Design review of the part built by this model. Coordinates are the model's own, in mm. A direction names the side the tool comes from. Coordinates: 2 decimals unless noted, no trailing zeros. Loops run counter-clockwise (first coordinate to the right, second up) from the corner with the lowest first, then second, coordinate; pieces in that order, holes last. Notation, with made-up numbers: (16.5, 39.5) - (71.5, 39.5) arc R32 cw to (71.5, 72.5) - close; hole circle Ø2 at (20, -33.75). An arc over 180 degrees is marked (long way). Answer in a Markdown table with one row per item. Add a question column.
(1) The part is to be moulded in two halves that separate along X. For faces 1 (the face through (-6.6, 24.02, -18.25)), 2 (the face through (-3.792, 14, -18)), 3 (the face through (-4, 28.312, -4)), say which applies: released by +X, released by -X, zero draft, split by the parting line, or undercut.
(2) We need section A-A, the plane y = 43. Write out the cut boundary in (x, z).
(3) We need section C-C, the plane x = 27.5. Write out the cut boundary in (y, z), plus the area to 3 significant figures.
(4) To check wall thickness, follow L1, parallel to X at y = 29, z = -18; L2, parallel to Z at x = 107, y = 11; L3, parallel to X at y = 46, z = -14. State the ranges of each line that lie inside material, in increasing order. Write a range as [from, to].
(5) Clearance check with flat-ended pins moving along their axes: pin 1 (12 mm diameter, centred on x = 22, z = -19.5, fed in from -Y); pin 2 (1 mm diameter, centred on y = 9, z = -18, fed in from -X); pin 3 (8 mm diameter, centred on y = 28.5, z = -17.5, fed in from +X); pin 4 (9.5 mm diameter, centred on x = 5.71, z = -18, fed in from +Y). State where each tip first meets the part, or that it passes through.
(6) We need section B-B, the plane x = 104. Write out the cut boundary in (y, z), plus the area to 3 significant figures.
(7) For faces 4 (the face through (-27, 22.312, -26)), 5 (the face through (3, 11, -28)), 6 (the face through (80, 28.312, -4)), 7 (the face through (93.71, 16.4, -17.89)), list the 3-axis set-ups (+Z, -Z, +X, -X, +Y, -Y) from which the entire face can be reached by the end or side of a thin tool; tool diameter is ignored.
from build123d import *

# Parameters (mm, degrees)
SKETCH1_W                = 168
SKETCH1_H                = 55
BOSS_EXTRUDE2_DEPTH      = 36
CUT_EXTRUDE2_DEPTH       = 41
CUT_EXTRUDE4_DEPTH       = 35
SKETCH5_W                = 44
SKETCH5_H                = 36
CUT_EXTRUDE5_DEPTH       = 12
CUT_EXTRUDE6_DEPTH       = 42
SKETCH11_R               = 5.25
CUT_EXTRUDE8_DEPTH       = 53
CUT_EXTRUDE9_DEPTH       = 46
FILLET1_R                = 6
SKETCH30_W               = 68
SKETCH30_H               = 20
CUT_EXTRUDE14_DEPTH      = 2
CUT_EXTRUDE16_DEPTH      = 6
CUT_EXTRUDE16_DEPTH_BACK = 6
SKETCH31_R               = 3
SKETCH32_W               = 20
SKETCH32_H               = 20
CUT_EXTRUDE19_DEPTH      = 7
CUT_EXTRUDE21_DEPTH      = 12


with BuildPart() as part:
    # Sketch1 → Boss-Extrude2 (new body)
    with BuildSketch(Plane.XY):
        with Locations((38.207905975, 35.811584747)):
            Rectangle(SKETCH1_W, SKETCH1_H)
    extrude(amount=-BOSS_EXTRUDE2_DEPTH)

    # Sketch3 → Cut-Extrude2 (cut)
    with BuildSketch(Plane(origin=(0, 63.311584747, 0), x_dir=(1, 0, 0), z_dir=(0, 1, 0))):
        Polygon((122.207905975, 36), (81.207905975, 36), (81.207905975, 18.000000234), (81.207905975, 0), (122.207905975, 0), align=None)
        Polygon((-4.792094025, 18), (-4.792094025, 36), (-45.792094025, 36), (-45.792094025, 0), (-4.792094025, 0), align=None)
    extrude(amount=-CUT_EXTRUDE2_DEPTH, mode=Mode.SUBTRACT)

    # Sketch4 → Cut-Extrude4 (cut)
    with BuildSketch(Plane(origin=(0, 63.311584747, 0), x_dir=(1, 0, 0), z_dir=(0, 1, 0))):
        with BuildLine():
            Line((-0.843342405, 36), (-4.792094025, 36))
            Line((-4.792094025, 36), (-4.792094025, 18))
            ThreePointArc((-4.792094025, 18), (-3.793306391, 27.214019744), (-0.843342405, 36))
        make_face()
        with BuildLine():
            ThreePointArc((-0.843342405, 0), (-3.793306391, 8.785980256), (-4.792094025, 18))
            Line((-4.792094025, 18), (-4.792094025, 0))
            Line((-4.792094025, 0), (-0.843342405, 0))
        make_face()
        with BuildLine():
            Line((81.207905975, 36), (77.259154354, 36))
            ThreePointArc((77.259154354, 36), (80.20911834, 27.214019744), (81.207905975, 18))
            Line((81.207905975, 18), (81.207905975, 36))
        make_face()
        with BuildLine():
            ThreePointArc((81.207905975, 18), (80.20911834, 8.785980256), (77.259154354, 0))
            Line((77.259154354, 0), (81.207905975, 0))
            Line((81.207905975, 0), (81.207905975, 18))
        make_face()
    extrude(amount=-CUT_EXTRUDE4_DEPTH, mode=Mode.SUBTRACT)

    # Sketch5 → Cut-Extrude5 (cut)
    with BuildSketch(Plane(origin=(0, 63.311584747, 0), x_dir=(1, 0, 0), z_dir=(0, 1, 0))):
        with Locations((38.207905975, 18)):
            Rectangle(SKETCH5_W, SKETCH5_H)
    extrude(amount=-CUT_EXTRUDE5_DEPTH, mode=Mode.SUBTRACT)

    # Sketch8 → Cut-Extrude6 (cut)
    with BuildSketch(Plane.XY):
        with BuildLine():
            ThreePointArc((19.446242935, 51.311584747), (36.703179712, 29.37126271), (57.207905975, 48.311584747))
            ThreePointArc((57.207905975, 48.311584747), (57.148228012, 49.81631101), (56.969569014, 51.311584747))
            Line((56.969569014, 51.311584747), (19.446242935, 51.311584747))
        make_face()
        with BuildLine():
            Line((19.446242935, 51.311584747), (56.969569014, 51.311584747))
            ThreePointArc((56.969569014, 51.311584747), (38.207905975, 67.311584747), (19.446242935, 51.311584747))
        make_face()
    extrude(amount=-CUT_EXTRUDE6_DEPTH, mode=Mode.SUBTRACT)

    # Sketch11 → Cut-Extrude8 (cut)
    with BuildSketch(Plane(origin=(0, 63.311584747, 0), x_dir=(1, 0, 0), z_dir=(0, 1, 0))):
        with Locations(Location((5.707905975, 18, 0), (0, 0, 270))):
            Circle(SKETCH11_R)
        with Locations(Location((70.707905975, 18, 0), (0, 0, 90))):
            Circle(SKETCH11_R)
    extrude(amount=-CUT_EXTRUDE8_DEPTH, mode=Mode.SUBTRACT)

    # Sketch13 → Cut-Extrude9 (cut)
    with BuildSketch(Plane.XY):
        Polygon((-45.792094025, 22.311584747), (-45.792094025, 8.311584747), (-41.792094025, 22.311584747), align=None)
        Polygon((122.207905975, 22.311584747), (118.207905975, 22.311584747), (122.207905975, 8.311584747), align=None)
    extrude(amount=-CUT_EXTRUDE9_DEPTH, mode=Mode.SUBTRACT)

    # Fillet1
    fillet1_edges = [part.edges().sort_by_distance(p)[0] for p in [
        (81.207905975, 22.311584747, -18),
        (-4.792094025, 22.311584747, -18),
    ]]
    fillet(fillet1_edges, radius=FILLET1_R - 0.0001)  # a hair under: the kernel refuses the full size

    # Sketch30 → Cut-Extrude14 (cut)
    with BuildSketch(Plane.XZ.offset(-8.311584747)):
        with Locations((-3.792094025, -18)):
            Rectangle(SKETCH30_W, SKETCH30_H)
        with Locations((80.207905975, -18)):
            Rectangle(SKETCH30_W, SKETCH30_H)
    extrude(amount=-CUT_EXTRUDE14_DEPTH, mode=Mode.SUBTRACT)

    # Sketch31 → Cut-Extrude16 (cut, two sides: drawn at the far end of the back side and taken through both)
    with BuildSketch(Plane(origin=(0, 29, 0), x_dir=(1, 0, 0), z_dir=(0, 1, 0)).offset(-CUT_EXTRUDE16_DEPTH_BACK)):
        with Locations(Location((38.207905975, 18, 0), (0, 0, 90))):
            Circle(SKETCH31_R)
    extrude(amount=CUT_EXTRUDE16_DEPTH + CUT_EXTRUDE16_DEPTH_BACK, mode=Mode.SUBTRACT)

    # Sketch32 → Cut-Extrude19 (cut)
    with BuildSketch(Plane.XZ.offset(-10.311584747)):
        with Locations((6.207905975, -18)):
            Rectangle(SKETCH32_W, SKETCH32_H)
        with Locations((71.078776846, -18)):
            Rectangle(SKETCH32_W, SKETCH32_H)
    extrude(amount=-CUT_EXTRUDE19_DEPTH, mode=Mode.SUBTRACT)

    # Sketch15 → Cut-Extrude21 (cut)
    with BuildSketch(Plane(origin=(0, 22.311584747, 0), x_dir=(1, 0, 0), z_dir=(0, 1, 0))):
        with BuildLine():
            Line((-30.292094025, 23), (-22.292094025, 23))
            ThreePointArc((-22.292094025, 23), (-17.292094025, 18), (-22.292094025, 13))
            Line((-22.292094025, 13), (-30.292094025, 13))
            ThreePointArc((-30.292094025, 13), (-35.292094025, 18), (-30.292094025, 23))
        make_face()
        with BuildLine():
            Line((98.707905975, 23), (106.707905975, 23))
            ThreePointArc((106.707905975, 23), (111.707905975, 18), (106.707905975, 13))
            Line((106.707905975, 13), (98.707905975, 13))
            ThreePointArc((98.707905975, 13), (93.707905975, 18), (98.707905975, 23))
        make_face()
    extrude(amount=-CUT_EXTRUDE21_DEPTH, mode=Mode.SUBTRACT)


solid = part.part
Responses:
| question | item | result |
|---|---|---|
| 1 | face 1 | released by -X |
| 1 | face 2 | undercut |
| 1 | face 3 | zero draft |
| 2 | outline | (-0.84, -36) - (19.97, -36) - (19.97, 0) - (-0.84, 0) arc R43 ccw to start; (56.45, -36) - (77.26, -36) arc R43 ccw to (77.26, 0) - (56.45, 0) - close; hole circle Ø10.5 at (5.71, -18); hole circle Ø10.5 at (70.71, -18) |
| 3 | outline | (8.31, -36) - (32.62, -36) - (32.62, 0) - (8.31, 0) - (8.31, -8) - (10.31, -8) - (10.31, -28) - (8.31, -28) - close |
| 3 | area | 835 mm2 |
| 4 | L1 | x = [-4.79, 0.46], [10.96, 35.21], [41.21, 65.46], [75.96, 81.21] |
| 4 | L2 | z = [-36, -22.99], [-13.01, 0] |
| 4 | L3 | x = [-4.61, 2.31], [9.11, 19.35], [57.07, 67.31], [74.11, 81.02] |
| 5 | pin 1 | stops at y = 10.31 |
| 5 | pin 2 | stops at x = -45.74 |
| 5 | pin 3 | stops at x = 82.57 |
| 5 | pin 4 | passes through |
| 6 | outline | (8.31, -36) - (22.31, -36) - (22.31, -23) - (10.31, -23) - (10.31, -28) - (8.31, -28) - close; (8.31, -8) - (10.31, -8) - (10.31, -13) - (22.31, -13) - (22.31, 0) - (8.31, 0) - close |
| 6 | area | 344 mm2 |
| 7 | face 4 | +Z, -Z, -X, +Y |
| 7 | face 5 | -Y |
| 7 | face 6 | +Z, +X, +Y |
| 7 | face 7 | +Y, -Y |
